Geometry: see drawing. Coordinates: mm, zero at the bounding-box minimum. A direction names the side the tool comes from. Give positions to 0.01 mm unless a question says otherwise; leave off trailing zeros. Order: outer loops, then holes, each group sorted by start corner. A loop starts at its lowest first (then second) coordinate and runs counter-clockwise, first axis right, second up. Notation, with made-up numbers: (-28, -0.5) - (12, -0.5) arc R19 ccw to (12, 33.5) - close; hole circle Ø5 at (-33, 61). An arc over 180 degrees is marked (long way). Write item = value, one per line. Start each with the question number.
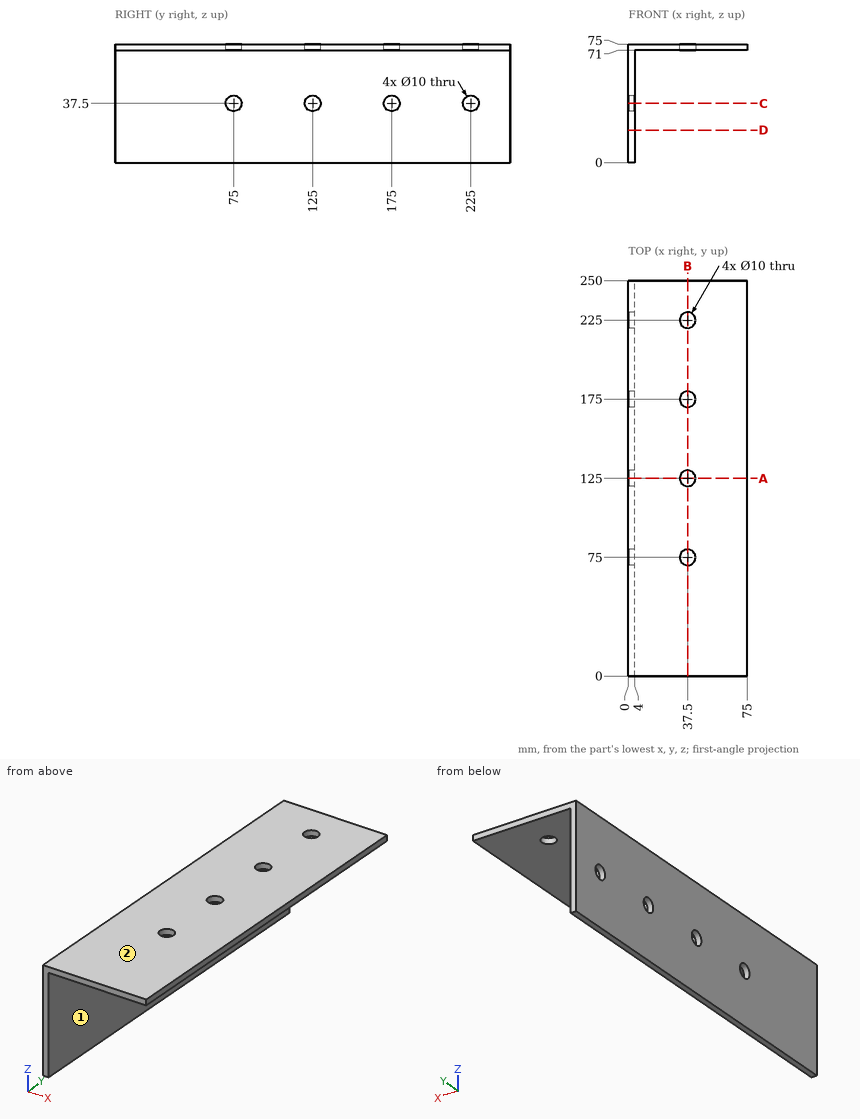
Q1. Section B-B, the plane x = 37.5. Return the cut outline in (y, z).
Q2. Section A-A, the plane y = 125. Return the cut outline in (x, z).
Q3. Section D-D, the plane z = 20.5. Return the cut outline in (x, y).
Q4. Section C-C, the plane z = 37.5. Return the cut outline in (x, y), then the cut area to 3 significant figures.
Q5. Material intervals for line 1 along Y through (x, z) = (37.5, 73.35); line 2 along X through (y, z) = (174, 49.5); line 3 along Z through (x, y) = (40, 104), sorted ascending. Write a range as from..to.
Q6. Contact query for flat-ended pins moving along their axis: pin 1 (21.5 mm diameter, centred on x = 38, y = 90.5, fed in from -Z); pin 2 (8 mm diameter, centred on y = 175, z = 37.5, fed in from +X); pin 3 (10 mm diameter, centred on y = 220, z = 35, fed in from +X). Output: stop coordinate, or through.
Q7. Set-up query: the marked faces 1 and 2. Return all of +Z, -Z, +X, -X, +Y, -Y with unobstructed straight access to the full face (end or side cutting, diameter ignored); none if empty.
The answers:
q1.outline = (0, 71) - (70, 71) - (70, 75) - (0, 75) - close; (80, 71) - (120, 71) - (120, 75) - (80, 75) - close; (130, 71) - (170, 71) - (170, 75) - (130, 75) - close; (180, 71) - (220, 71) - (220, 75) - (180, 75) - close; (230, 71) - (250, 71) - (250, 75) - (230, 75) - close
q2.outline = (0, 0) - (4, 0) - (4, 32.5) - (0, 32.5) - close; (0, 42.5) - (4, 42.5) - (4, 71) - (32.5, 71) - (32.5, 75) - (0, 75) - close; (42.5, 71) - (75, 71) - (75, 75) - (42.5, 75) - close
q3.outline = (0, 0) - (4, 0) - (4, 250) - (0, 250) - close
q4.outline = (0, 0) - (4, 0) - (4, 70) - (0, 70) - close; (0, 80) - (4, 80) - (4, 120) - (0, 120) - close; (0, 130) - (4, 130) - (4, 170) - (0, 170) - close; (0, 180) - (4, 180) - (4, 220) - (0, 220) - close; (0, 230) - (4, 230) - (4, 250) - (0, 250) - close
q4.area = 840 mm²
q5.line_1 = 0..70, 80..120, 130..170, 180..220, 230..250
q5.line_2 = 0..4
q5.line_3 = 71..75
q6.pin_1 = 71
q6.pin_2 = through
q6.pin_3 = 4
q7.face_1 = -Z, +X, +Y, -Y
q7.face_2 = +Z, +X, -X, +Y, -Y
